from build123d import *

# Parameters (mm, degrees)
SKETCH_1_W          = 10
SKETCH_1_H          = 10
SKETCH_1_W_2        = 8
SKETCH_1_H_2        = 8
EXTRUDE_1_DEPTH     = 100
SKETCH_3_R          = 1.5
CUT_EXTRUDE_2_DEPTH = 101.623058987
SKETCH_4_R          = 1.5
SKETCH_4_R_2        = 2
CUT_EXTRUDE_3_DEPTH = 101.623058987
SKETCH_5_W          = 10
SKETCH_5_H          = 10
SKETCH_5_W_2        = 8
SKETCH_5_H_2        = 8
EXTRUDE_2_DEPTH     = 10
SKETCH_6_R          = 1.5
CUT_EXTRUDE_4_DEPTH = 101.623058987


with BuildPart() as part:
    # ｽｹｯﾁ1 → 押し出し-薄板1 (new body)
    with BuildSketch(Plane.XY):
        Rectangle(SKETCH_1_W, SKETCH_1_H)
        Rectangle(SKETCH_1_W_2, SKETCH_1_H_2, mode=Mode.SUBTRACT)
    extrude(amount=EXTRUDE_1_DEPTH)

    # ｽｹｯﾁ3 → ｶｯﾄ - 押し出し2 (cut, through all)
    with BuildSketch(Plane.XZ.offset(5)):
        with Locations((0, 15)):
            Circle(SKETCH_3_R)
        with Locations((0, 85)):
            Circle(SKETCH_3_R)
    extrude(amount=-CUT_EXTRUDE_2_DEPTH, mode=Mode.SUBTRACT)

    # ｽｹｯﾁ4 → ｶｯﾄ - 押し出し3 (cut, through all)
    with BuildSketch(Plane(origin=(5, 0, 0), x_dir=(0, 0, -1), z_dir=(1, 0, 0))):
        with Locations((-64.61, 0)):
            Circle(SKETCH_4_R)
        with Locations(Location((-35.39, 0, 0), (0, 0, 180))):
            Circle(SKETCH_4_R)
        with Locations(Location((-95, 0, 0), (0, 0, 180))):
            Circle(SKETCH_4_R_2)
    extrude(amount=-CUT_EXTRUDE_3_DEPTH, mode=Mode.SUBTRACT)

    # ｽｹｯﾁ5 → 押し出し-薄板2 (add)
    with BuildSketch(Plane(origin=(0, 0, 0), x_dir=(-1, 0, 0), z_dir=(0, 0, -1))):
        Rectangle(SKETCH_5_W, SKETCH_5_H)
        Rectangle(SKETCH_5_W_2, SKETCH_5_H_2, mode=Mode.SUBTRACT)
    extrude(amount=EXTRUDE_2_DEPTH)

    # ｽｹｯﾁ6 → ｶｯﾄ - 押し出し4 (cut, through all)
    with BuildSketch(Plane(origin=(0, 5, 0), x_dir=(1, 0, 0), z_dir=(0, 1, 0))):
        with Locations(Location((0, 5, 0), (0, 0, 180))):
            Circle(SKETCH_6_R)
    extrude(amount=-CUT_EXTRUDE_4_DEPTH, mode=Mode.SUBTRACT)


solid = part.part
Can you work these out from the model? Positions are in its coordinate system, mm. A direction names the side the tool comes from. Coordinates: 2 decimals unless noted, no trailing zeros. Order: outer loops, then holes, each group sorted by start corner. A loop starts at its lowest first (then second) coordinate and runs counter-clockwise, first axis right, second up. Notation, with made-up numbers: M -9,56.5 L 10,56.5 A4 ccw 10,63.5 Z; hole C 24.5,-35.5 d8. An arc over 180 degrees is marked long. Answer as CSV lines item,"result".
(1) Suppose I cut it at A-A on y = 0. Count the separate pieces of the cut face and the enclosed holes in it, plus the area to 3 significant figures.
Geometry check:
separate pieces,"8"
enclosed holes,"0"
area,"200 mm^2"
(2) On a 3-axis mill with a long thin cutter (end or side, diameter ignored), from which of +Z, -Z, +X, -X, +Y, -Y can I reach the whole of each face in a straight line? I mean faces 4 (the flat face through (-4, 0, 46)), 5 (the flat face through (-5, 0, 46)). Say none if no direction works.
Geometry check:
face 4,"+Z, -Z"
face 5,"+Z, -Z, -X, +Y, -Y"
(3) Suppose I cut it at D-D on z = 35.39. Please give me the cut outline in (x, y).
Geometry check:
outline,"M -5,-5 L 5,-5 L 5,-1.5 L 4,-1.5 L 4,-4 L -4,-4 L -4,-1.5 L -5,-1.5 Z; M -5,1.5 L -4,1.5 L -4,4 L 4,4 L 4,1.5 L 5,1.5 L 5,5 L -5,5 Z"
(4) Please list where these lines run through material, in increasing order: L1, parallel to Z at x = 0, y = 4.7; L2, parallel to Y at x = -1, z = 37.
Geometry check:
L1,"-10 to -6.5, -3.5 to 13.5, 16.5 to 83.5, 86.5 to 100"
L2,"-5 to -4, 4 to 5"
(5) Suppose I cut it at B-B on z = 57.5. Please give me the cut outline in (x, y), plus the area to 3 significant figures.
Geometry check:
outline,"M -5,-5 L 5,-5 L 5,5 L -5,5 Z; hole M -4,-4 L 4,-4 L 4,4 L -4,4 Z"
area,"36.0 mm^2"
(6) If we mould it in two halves opening along X, with no side actions, what happens to faces 1 (the flat face through (0, 4, 46)), 2 (the flat face through (5, 0, 46)), 3 (the cylindrical face through (-4.493, -0.601, 96.908))? For each: released by +X, released by -X, zero draft, split by the parting line, or undercut.
Geometry check:
face 1,"undercut"
face 2,"released by +X"
face 3,"zero draft"
